```python
from build123d import *

# Parameters (mm, degrees)
SKETCH1_W                      = 28
SKETCH1_H                      = 10
BOSS_EXTRUDE1_DEPTH            = 5
SKETCH6_R                      = 6
BOSS_EXTRUDE3_DEPTH            = 9
BOSS_EXTRUDE4_DEPTH            = 4.5
CUT_EXTRUDE1_DEPTH             = 87.075548212
CUT_EXTRUDE1_DEPTH_BACK        = 87.075548212
SKETCH8_R                      = 2
CUT_EXTRUDE2_DEPTH             = 85.65222974
CUT_EXTRUDE2_DEPTH_BACK        = 85.65222974
CUT_EXTRUDE3_REACH             = 88.076
SKETCH10_R                     = 3
CUT_EXTRUDE3_DIRECTION_2_DEPTH = 87.075548212
CUT_EXTRUDE4_REACH             = 76.873
SKETCH11_R                     = 2
FILLET1_R                      = 1
FILLET2_R                      = 1
CUT_EXTRUDE5_DEPTH             = 85.65222974
CUT_EXTRUDE5_DEPTH_BACK        = 85.65222974


with BuildPart() as part:
    # Sketch1 → Boss-Extrude1 (new, symmetric)
    with BuildSketch(Plane.XY):
        with Locations((0, 5)):
            Rectangle(SKETCH1_W, SKETCH1_H)
    extrude(amount=BOSS_EXTRUDE1_DEPTH, both=True)

    # Sketch2 → Revolve2 (revolve)
    with BuildSketch(Plane(origin=(0, 0, 0), x_dir=(0, 0, -1), z_dir=(1, 0, 0)), mode=Mode.PRIVATE) as revolve2_sk:
        Polygon((0, 10), (0, 77), (-4, 77), (-4.5, 10), align=None)
    revolve(revolve2_sk.sketch.rotate(Axis((0, 10, 0), (0, 1, 0)), 180), axis=Axis((0, 10, 0), (0, 1, 0)))

    # Sketch6 → Boss-Extrude3 (add, symmetric)
    with BuildSketch(Plane.XY):
        with Locations((0, 77)):
            Circle(SKETCH6_R)
    extrude(amount=BOSS_EXTRUDE3_DEPTH, both=True)

    # Sketch7 → Boss-Extrude4 (add, symmetric)
    with BuildSketch(Plane(origin=(0, 0, 0), x_dir=(0, 0, -1), z_dir=(1, 0, 0))):
        with BuildLine():
            Line((-8, 77), (8, 77))
            Line((8, 77), (8, 68))
            ThreePointArc((8, 68), (0, 60), (-8, 68))
            Line((-8, 68), (-8, 77))
        make_face()
    extrude(amount=BOSS_EXTRUDE4_DEPTH, both=True)

    # Sketch8 → Cut-Extrude1 (cut, two sides: drawn at the far end of the back side and taken through both)
    with BuildSketch(Plane.XY.offset(9).offset(-CUT_EXTRUDE1_DEPTH_BACK)):
        with Locations((0, 77)):
            Circle(SKETCH8_R)
    extrude(amount=CUT_EXTRUDE1_DEPTH + CUT_EXTRUDE1_DEPTH_BACK, mode=Mode.SUBTRACT)

    # Sketch9 → Cut-Extrude2 (cut, two sides: drawn at the far end of the back side and taken through both)
    with BuildSketch(Plane(origin=(0, 0, 0), x_dir=(0, 0, -1), z_dir=(1, 0, 0)).offset(-CUT_EXTRUDE2_DEPTH_BACK)):
        with BuildLine():
            Line((-4.5, 68), (-4.5, 86.268805497))
            ThreePointArc((-4.5, 86.268805497), (0, 90.768805497), (4.5, 86.268805497))
            Line((4.5, 86.268805497), (4.5, 68))
            ThreePointArc((4.5, 68), (0, 63.5), (-4.5, 68))
        make_face()
    extrude(amount=CUT_EXTRUDE2_DEPTH + CUT_EXTRUDE2_DEPTH_BACK, mode=Mode.SUBTRACT)

    # Sketch10 → Cut-Extrude3 (cut, up to next)
    with BuildSketch(Plane.XY.offset(9), mode=Mode.PRIVATE) as cut_extrude3_sk1:
        with Locations((0, 77)):
            Circle(SKETCH10_R)
    cut_extrude3_tool1 = extrude(cut_extrude3_sk1.sketch, amount=-CUT_EXTRUDE3_REACH, mode=Mode.PRIVATE) & part.part
    add(cut_extrude3_tool1.solids().sort_by_distance((0, 77, 9))[0], mode=Mode.SUBTRACT)

    # Sketch10 → Cut-Extrude3 direction 2 (cut)
    with BuildSketch(Plane.XY.offset(9)):
        with Locations((0, 77)):
            Circle(SKETCH10_R)
    extrude(amount=CUT_EXTRUDE3_DIRECTION_2_DEPTH, mode=Mode.SUBTRACT)

    # Sketch11 → Cut-Extrude4 (cut, up to next)
    with BuildSketch(Plane(origin=(0, 10, 0), x_dir=(1, 0, 0), z_dir=(0, 1, 0)), mode=Mode.PRIVATE) as cut_extrude4_sk1:
        with Locations(Location((-10, 0, 0), (0, 0, 270))):
            Circle(SKETCH11_R)
    cut_extrude4_tool1 = extrude(cut_extrude4_sk1.sketch, amount=-CUT_EXTRUDE4_REACH, mode=Mode.PRIVATE) & part.part
    # Sketch11 → Cut-Extrude4 (cut, up to next)
    with BuildSketch(Plane(origin=(0, 10, 0), x_dir=(1, 0, 0), z_dir=(0, 1, 0)), mode=Mode.PRIVATE) as cut_extrude4_sk2:
        with Locations(Location((10, 0, 0), (0, 0, 270))):
            Circle(SKETCH11_R)
    cut_extrude4_tool2 = extrude(cut_extrude4_sk2.sketch, amount=-CUT_EXTRUDE4_REACH, mode=Mode.PRIVATE) & part.part
    add(cut_extrude4_tool1.solids().sort_by_distance((-10, 10, 0))[0], mode=Mode.SUBTRACT)
    add(cut_extrude4_tool2.solids().sort_by_distance((10, 10, 0))[0], mode=Mode.SUBTRACT)

    # Fillet1
    fillet1_edges = [part.edges().sort_by_distance(p)[0] for p in [
        (14, 5, 5),
        (-14, 5, 5),
        (14, 5, -5),
        (-14, 5, -5),
    ]]
    fillet(fillet1_edges, radius=FILLET1_R)

    # Fillet2
    fillet2_edges = [part.edges().sort_by_distance(p)[0] for p in [
        (0, 10, 4.5),
    ]]
    fillet(fillet2_edges, radius=FILLET2_R)

    # Sketch12 → Cut-Extrude5 (cut, two sides: drawn at the far end of the back side and taken through both)
    with BuildSketch(Plane.XY.offset(-CUT_EXTRUDE5_DEPTH_BACK)):
        with BuildLine():
            Line((-6.5, 0), (6.5, 0))
            ThreePointArc((6.5, 0), (0, 6.5), (-6.5, 0))
        make_face()
    extrude(amount=CUT_EXTRUDE5_DEPTH + CUT_EXTRUDE5_DEPTH_BACK, mode=Mode.SUBTRACT)


solid = part.part
```
The listing builds one solid part. Answer for the finished solid, in the listing's coordinates (mm). A direction names the side the tool comes from. Round coordinates to 2 decimals unless told otherwise and drop trailing zeros. Loops run counter-clockwise (first coordinate to the right, second up) from the corner with the lowest first, then second, coordinate; pieces in that order, holes last. Notation, with made-up numbers: (57.5, 66.25) -> (96.5, 66.25) arc R16 cw to (96.5, 85.25) -> close; hole circle Ø2 at (43, -15). An arc over 180 degrees is marked (long way). Use one line per item in the form item = value.
1. The part is cut by section B-B on y = 77. Determine the outline of the cut face in (x, z), and give its area (3 significant figures).
Answer key:
outline = (-6, -9) -> (-2, -9) -> (-2, -4.5) -> (-6, -4.5) -> close; (-6, 4.5) -> (-3, 4.5) -> (-3, 9) -> (-6, 9) -> close; (2, -9) -> (6, -9) -> (6, -4.5) -> (2, -4.5) -> close; (3, 4.5) -> (6, 4.5) -> (6, 9) -> (3, 9) -> close
area = 63.0 mm²
2. Flat-ended cylindrical pins translate along their axes: pin 1 Ø4 at (y, z) = (67.5, -2) entering from +X; pin 2 Ø6 at (y, z) = (70, 2) entering from +X; pin 3 Ø4 at (x, z) = (-8, 1.5) entering from +Y; pin 4 Ø11 at (x, y) = (6, 6.5) entering from -Z. Find the tip coordinate at first contact, or state that the pin passes through.
Answer key:
pin_1 = through
pin_2 = 4.5
pin_3 = 10
pin_4 = -5
3. The part is cut by section C-C on z = 5.75. Determine the outline of the cut face in (x, y), and give its area (3 significant figures).
Answer key:
outline = (-4.5, 62.44) -> (4.5, 62.44) -> (4.5, 73.03) arc R6 ccw (long way) to (-4.5, 73.03) -> close; hole circle Ø6 at (0, 77)
area = 167 mm²
4. A tool of negligible diameter and unlimited length cuts with its end or side. For faces 1 (the flat face through (0, 7, -5)), 2 (the flat face through (-4.5, 63.7, -1.9)), 3 (the flat face through (4.5, 63.7, -1.9)), 4 (the flat face through (0, 7, 5)), from which of +Z, -Z, +X, -X, +Y, -Y can it reach the whole face along a straight path? Write none if from no direction.
Answer key:
face_1 = -Z, +X, -X, -Y
face_2 = +Z, -Z, -X
face_3 = +Z, -Z, +X
face_4 = +Z, +X, -X, -Y
5. The part is cut by section A-A on x = 10. Determine the outline of the cut face in (y, z).
Answer key:
outline = (0, -5) -> (10, -5) -> (10, -2) -> (0, -2) -> close; (0, 2) -> (10, 2) -> (10, 5) -> (0, 5) -> close
6. Find the intervals of material crossed by probe 1 along X at (y, z) = (2.5, 0); probe 2 along X at (y, z) = (7.25, 0); probe 3 along X at (y, z) = (7, 1.75), in increasing order. Write a range as [from, to].
Answer key:
probe_1 = [-14, -12], [-8, -6], [6, 8], [12, 14]
probe_2 = [-14, -12], [-8, 8], [12, 14]
probe_3 = [-14, -10.97], [-9.03, 9.03], [10.97, 14]
7. For a pull along Z with two mould halves and no side action, classify faces 5 (the flat face through (-3, 76, 9)), 6 (the conical face through (-1.29, 35.63, -4.11)), 7 (the flat face through (0, 74, -4.5)) as released by +Z, released by -Z, zero draft, split by the parting line, or undercut.
Answer key:
face_5 = released by +Z
face_6 = split by the parting line
face_7 = undercut
8. The part is cut by section D-D on x = -11. Determine the outline of the cut face in (y, z).
Answer key:
outline = (0, -5) -> (10, -5) -> (10, -1.73) -> (0, -1.73) -> close; (0, 1.73) -> (10, 1.73) -> (10, 5) -> (0, 5) -> close
